```python
from build123d import *

# Parameters (mm, degrees)
SKETCH1_R           = 5.7
BOSS_EXTRUDE1_DEPTH = 8
SKETCH2_R           = 5.25
BOSS_EXTRUDE2_DEPTH = 16.5
SKETCH3_R           = 8.5
BOSS_EXTRUDE3_DEPTH = 6.6
BOSS_EXTRUDE3_TAPER = 13
SKETCH4_R           = 5.9
BOSS_EXTRUDE4_DEPTH = 3.7


with BuildPart() as part:
    # Sketch1 → Boss-Extrude1 (new body)
    with BuildSketch(Plane(origin=(0, 0, 0), x_dir=(1, 0, 0), z_dir=(0, 1, 0))):
        with Locations(Location((0, 0, 0), (0, 0, 270))):  # turned: the seam where the file's is
            Circle(SKETCH1_R)
    extrude(amount=BOSS_EXTRUDE1_DEPTH)

    # Sketch2 → Boss-Extrude2 (add)
    with BuildSketch(Plane(origin=(0, 8, 0), x_dir=(1, 0, 0), z_dir=(0, 1, 0))):
        with Locations(Location((0, 0, 0), (0, 0, 270))):  # turned: the seam where the file's is
            Circle(SKETCH2_R)
    extrude(amount=BOSS_EXTRUDE2_DEPTH)

    # Sketch3 → Boss-Extrude3 (add)
    with BuildSketch(Plane.XZ):
        Circle(SKETCH3_R)
    extrude(amount=BOSS_EXTRUDE3_DEPTH, taper=BOSS_EXTRUDE3_TAPER)

    # Sketch4 → Boss-Extrude4 (add)
    with BuildSketch(Plane.XZ.offset(6.6)):
        with Locations(Location((0, 0, 0), (0, 0, 270))):  # turned: the seam where the file's is
            Circle(SKETCH4_R)
    extrude(amount=BOSS_EXTRUDE4_DEPTH)


solid = part.part
```
Design review of the part built by this model. Coordinates are the model's own, in mm. A direction names the side the tool comes from. Give positions to 0.01 mm unless a question says otherwise; leave off trailing zeros. Write each loop counter-clockwise with the first axis right and the second up, starting at its lowest first coordinate (ties: lowest second). Pieces come first, ordered by that corner, then holes. Notation, with made-up numbers: (-17.5, 29) -> (21.5, 29) arc R20 cw to (21.5, 44) -> close; hole circle Ø5 at (-33.5, 0). An arc over 180 degrees is marked (long way). Answer in a Markdown table with one row per item.
(1) Consider section C-C (y = -6). State the section outline as (x, z) points.
Results:
| item | result |
|---|---|
| outline | circle Ø14.23 at (0, 0) |
(2) Consider section A-A (x = 0). State the section outline as (y, z) points, then the cut area to 3 significant figures.
Results:
| item | result |
|---|---|
| outline | (-10.3, -5.9) -> (-6.6, -5.9) -> (-6.6, -6.98) -> (0, -8.5) -> (0, -5.7) -> (8, -5.7) -> (8, -5.25) -> (24.5, -5.25) -> (24.5, 5.25) -> (8, 5.25) -> (8, 5.7) -> (0, 5.7) -> (0, 8.5) -> (-6.6, 6.98) -> (-6.6, 5.9) -> (-10.3, 5.9) -> close |
| area | 410 mm2 |
(3) For faces 1 (the flat face through (0, -10.3, 0)), 2 (the cylindrical face through (-5.76, -8.42, 1.28)), 3 (the flat face through (2, 0, -6)), list the 3-axis set-ups (+Z, -Z, +X, -X, +Y, -Y) from which the entire face can be reached by the end or side of a thin tool; tool diameter is ignored.
Results:
| item | result |
|---|---|
| face 1 | +Z, -Z, +X, -X, -Y |
| face 2 | -Y |
| face 3 | +Y |
(4) Clearance check with flat-ended pins moving along their axes: pin 1 (1.5 mm diameter, centred on y = 10.5, z = 0.5, fed in from +X); pin 2 (2 mm diameter, centred on x = 0, y = 11, fed in from +Z). State where each tip first meets the part, or that it passes through.
Results:
| item | result |
|---|---|
| pin 1 | x = 5.25 |
| pin 2 | z = 5.25 |
(5) Consider section B-B (y = 16.5). State the section outline as (x, z) points, then the cut area to 3 significant figures.
Results:
| item | result |
|---|---|
| outline | circle Ø10.5 at (0, 0) |
| area | 86.6 mm2 |
(6) To check wall thickness, follow probe 1 along Y at (x, z) = (3.75, -4.5); probe 2 along Y at (x, z) = (5.75, -3); probe 3 along X at (y, z) = (23, 0). State the ranges of each line that lie inside material, in increasing order.
Results:
| item | result |
|---|---|
| probe 1 | -10.3 to 0 |
| probe 2 | -6.6 to 0 |
| probe 3 | -5.25 to 5.25 |
